from build123d import *

# Parameters (mm, degrees)
F0_R      = 4
F1_DEPTH  = 0.8
F2_R      = 2.3
F3_DEPTH  = 4.5
F4_R      = 4.5
F5_DEPTH  = 13
F6_R      = 1.5
F7_DEPTH  = 9.4
F8_R      = 1.05
F9_DEPTH  = 12.5
F10_W     = 0.4
F10_H     = 0.6
F11_DEPTH = 25
F12_COUNT = 30
F15_DEPTH = 2.5


with BuildPart() as f1:
    # F0 (on Top) → F1 (new body)
    with BuildSketch(Plane.XY):
        Circle(F0_R)
    extrude(amount=F1_DEPTH)

    # F2 (on face) → F3 (join)
    with BuildSketch(Plane.XY.offset(0.8)):
        Circle(F2_R)
    extrude(amount=F3_DEPTH)

    # F4 (on face) → F5 (join)
    with BuildSketch(Plane.XY.offset(5.3)):
        Circle(F4_R)
    extrude(amount=F5_DEPTH)

    # F6 (on face) → F7 (join)
    with BuildSketch(Plane(origin=(0, 0, 0), x_dir=(1, 0, 0), z_dir=(0, 0, -1))):
        Circle(F6_R)
    extrude(amount=F7_DEPTH)

    # F8 (on Front) → F9 (cut, symmetric)
    with BuildSketch(Plane.XZ):
        with Locations((0, 3)):
            Circle(F8_R)
    extrude(amount=F9_DEPTH, both=True, mode=Mode.SUBTRACT)


with BuildPart() as f11:
    # F10 (on face) → F11 (new body)
    with BuildSketch(Plane.XY.offset(18.3)):
        with Locations((0, 4.5)):
            Rectangle(F10_W, F10_H)
    extrude(amount=-F11_DEPTH)


with BuildPart() as f12_1:
    # F12: instance of F11
    add(f11.part.rotate(Axis((0, 0, 18.3), (0, 0, 1)), 1 * 360 / F12_COUNT))


with BuildPart() as f12_2:
    # F12: instance of F11
    add(f11.part.rotate(Axis((0, 0, 18.3), (0, 0, 1)), 2 * 360 / F12_COUNT))


with BuildPart() as f12_3:
    # F12: instance of F11
    add(f11.part.rotate(Axis((0, 0, 18.3), (0, 0, 1)), 3 * 360 / F12_COUNT))


with BuildPart() as f12_4:
    # F12: instance of F11
    add(f11.part.rotate(Axis((0, 0, 18.3), (0, 0, 1)), 4 * 360 / F12_COUNT))


with BuildPart() as f12_5:
    # F12: instance of F11
    add(f11.part.rotate(Axis((0, 0, 18.3), (0, 0, 1)), 5 * 360 / F12_COUNT))


with BuildPart() as f12_6:
    # F12: instance of F11
    add(f11.part.rotate(Axis((0, 0, 18.3), (0, 0, 1)), 6 * 360 / F12_COUNT))


with BuildPart() as f12_7:
    # F12: instance of F11
    add(f11.part.rotate(Axis((0, 0, 18.3), (0, 0, 1)), 7 * 360 / F12_COUNT))


with BuildPart() as f12_8:
    # F12: instance of F11
    add(f11.part.rotate(Axis((0, 0, 18.3), (0, 0, 1)), 8 * 360 / F12_COUNT))


with BuildPart() as f12_9:
    # F12: instance of F11
    add(f11.part.rotate(Axis((0, 0, 18.3), (0, 0, 1)), 9 * 360 / F12_COUNT))


with BuildPart() as f12_10:
    # F12: instance of F11
    add(f11.part.rotate(Axis((0, 0, 18.3), (0, 0, 1)), 10 * 360 / F12_COUNT))


with BuildPart() as f12_11:
    # F12: instance of F11
    add(f11.part.rotate(Axis((0, 0, 18.3), (0, 0, 1)), 11 * 360 / F12_COUNT))


with BuildPart() as f12_12:
    # F12: instance of F11
    add(f11.part.rotate(Axis((0, 0, 18.3), (0, 0, 1)), 12 * 360 / F12_COUNT))


with BuildPart() as f12_13:
    # F12: instance of F11
    add(f11.part.rotate(Axis((0, 0, 18.3), (0, 0, 1)), 13 * 360 / F12_COUNT))


with BuildPart() as f12_14:
    # F12: instance of F11
    add(f11.part.rotate(Axis((0, 0, 18.3), (0, 0, 1)), 14 * 360 / F12_COUNT))


with BuildPart() as f12_15:
    # F12: instance of F11
    add(f11.part.rotate(Axis((0, 0, 18.3), (0, 0, 1)), 15 * 360 / F12_COUNT))


with BuildPart() as f12_16:
    # F12: instance of F11
    add(f11.part.rotate(Axis((0, 0, 18.3), (0, 0, 1)), 16 * 360 / F12_COUNT))


with BuildPart() as f12_17:
    # F12: instance of F11
    add(f11.part.rotate(Axis((0, 0, 18.3), (0, 0, 1)), 17 * 360 / F12_COUNT))


with BuildPart() as f12_18:
    # F12: instance of F11
    add(f11.part.rotate(Axis((0, 0, 18.3), (0, 0, 1)), 18 * 360 / F12_COUNT))


with BuildPart() as f12_19:
    # F12: instance of F11
    add(f11.part.rotate(Axis((0, 0, 18.3), (0, 0, 1)), 19 * 360 / F12_COUNT))


with BuildPart() as f12_20:
    # F12: instance of F11
    add(f11.part.rotate(Axis((0, 0, 18.3), (0, 0, 1)), 20 * 360 / F12_COUNT))


with BuildPart() as f12_21:
    # F12: instance of F11
    add(f11.part.rotate(Axis((0, 0, 18.3), (0, 0, 1)), 21 * 360 / F12_COUNT))


with BuildPart() as f12_22:
    # F12: instance of F11
    add(f11.part.rotate(Axis((0, 0, 18.3), (0, 0, 1)), 22 * 360 / F12_COUNT))


with BuildPart() as f12_23:
    # F12: instance of F11
    add(f11.part.rotate(Axis((0, 0, 18.3), (0, 0, 1)), 23 * 360 / F12_COUNT))


with BuildPart() as f12_24:
    # F12: instance of F11
    add(f11.part.rotate(Axis((0, 0, 18.3), (0, 0, 1)), 24 * 360 / F12_COUNT))


with BuildPart() as f12_25:
    # F12: instance of F11
    add(f11.part.rotate(Axis((0, 0, 18.3), (0, 0, 1)), 25 * 360 / F12_COUNT))


with BuildPart() as f12_26:
    # F12: instance of F11
    add(f11.part.rotate(Axis((0, 0, 18.3), (0, 0, 1)), 26 * 360 / F12_COUNT))


with BuildPart() as f12_27:
    # F12: instance of F11
    add(f11.part.rotate(Axis((0, 0, 18.3), (0, 0, 1)), 27 * 360 / F12_COUNT))


with BuildPart() as f12_28:
    # F12: instance of F11
    add(f11.part.rotate(Axis((0, 0, 18.3), (0, 0, 1)), 28 * 360 / F12_COUNT))


with BuildPart() as f12_29:
    # F12: instance of F11
    add(f11.part.rotate(Axis((0, 0, 18.3), (0, 0, 1)), 29 * 360 / F12_COUNT))


with BuildPart() as f1_1:
    add(f1.part)

    # F13: cut F12_1, F12_2, F12_3, F12_4, F12_5, F12_6, F12_7, F12_8, F12_9, F12_10, F12_11, F12_12, F12_13, F12_14, F12_15, F12_16, F12_17, F12_18, F12_19, F12_20, F12_21, F12_22, F12_23, F12_24, F12_25, F12_26, F12_27, F12_28, F12_29, F11
    add(f12_1.part, mode=Mode.SUBTRACT)
    add(f12_2.part, mode=Mode.SUBTRACT)
    add(f12_3.part, mode=Mode.SUBTRACT)
    add(f12_4.part, mode=Mode.SUBTRACT)
    add(f12_5.part, mode=Mode.SUBTRACT)
    add(f12_6.part, mode=Mode.SUBTRACT)
    add(f12_7.part, mode=Mode.SUBTRACT)
    add(f12_8.part, mode=Mode.SUBTRACT)
    add(f12_9.part, mode=Mode.SUBTRACT)
    add(f12_10.part, mode=Mode.SUBTRACT)
    add(f12_11.part, mode=Mode.SUBTRACT)
    add(f12_12.part, mode=Mode.SUBTRACT)
    add(f12_13.part, mode=Mode.SUBTRACT)
    add(f12_14.part, mode=Mode.SUBTRACT)
    add(f12_15.part, mode=Mode.SUBTRACT)
    add(f12_16.part, mode=Mode.SUBTRACT)
    add(f12_17.part, mode=Mode.SUBTRACT)
    add(f12_18.part, mode=Mode.SUBTRACT)
    add(f12_19.part, mode=Mode.SUBTRACT)
    add(f12_20.part, mode=Mode.SUBTRACT)
    add(f12_21.part, mode=Mode.SUBTRACT)
    add(f12_22.part, mode=Mode.SUBTRACT)
    add(f12_23.part, mode=Mode.SUBTRACT)
    add(f12_24.part, mode=Mode.SUBTRACT)
    add(f12_25.part, mode=Mode.SUBTRACT)
    add(f12_26.part, mode=Mode.SUBTRACT)
    add(f12_27.part, mode=Mode.SUBTRACT)
    add(f12_28.part, mode=Mode.SUBTRACT)
    add(f12_29.part, mode=Mode.SUBTRACT)
    add(f11.part, mode=Mode.SUBTRACT)

    # F14 (on face) → F15 (join)
    with BuildSketch(Plane(origin=(0, 0, 0), x_dir=(1, 0, 0), z_dir=(0, 0, -1))):
        Polygon((-2.6927305179, -0.8780481684), (-0.5859532394, -2.7709971182), (2.1067772785, -1.8929489498), (2.6927305179, 0.8780481684), (0.5859532394, 2.7709971182), (-2.1067772785, 1.8929489498), align=None)
    extrude(amount=F15_DEPTH)


solid = f1_1.part
Can you work these out from the model? Positions are in its coordinate system, mm. A direction names the side the tool comes from. Give positions to 0.01 mm unless a question says otherwise; leave off trailing zeros. Order: outer loops, then holes, each group sorted by start corner. A loop starts at its lowest first (then second) coordinate and runs counter-clockwise, first axis right, second up. Notation, with made-up numbers: M -30,28 L -3,28 A12 ccw -3,50 Z; hole C 20.25,25 d5. An arc over 180 degrees is marked long. Use one line per item in the form item = value.
Item 1: If I drill on line 1 along Z through (x, y) = (0, 0.2); line 2 along X through (y, z) = (0.1, 3); line 3 along Z through (x, y) = (3.75, 1), over which ranges is the centre line in solid material (lowest first)? Write a range as [from, to].
Values follow:
line_1 = [-9.4, 1.95], [4.05, 18.3]
line_2 = [-2.3, -1.05], [1.05, 2.3]
line_3 = [0, 0.8], [5.3, 18.3]
Item 2: If we section it at C-C, the plane z = -7: Write out the boundary of the cut face in (x, y), and give its area (3 significant figures).
Values follow:
outline = C 0,0 d3
area = 7.07 mm^2
Item 3: If we section it at B-B, the plane z = 3: Write out the boundary of the cut face in (x, y).
Values follow:
outline = M -1.05,-2.05 L -1.05,2.05 A2.3 ccw Z; M 1.05,-2.05 A2.3 ccw 1.05,2.05 Z
Item 4: Thinking about a two-plate mould opening in X: for faces 1 (the flat face through (1.654, -1.811, -1.232)), 2 (the flat face through (1.2, 1.2, -2.5)), 3 (the cylindrical face through (0.485, -0.032, 2.068)), which applies, pulls with the +X half, pulls with the -X half, needs draft (parallel to the pull), parting line crosses it, or undercut?
Values follow:
face_1 = pulls with the +X half
face_2 = needs draft
face_3 = undercut
Item 5: Will these pins go through, and if not, where does the flat tip stop? pin 1 Ø1.7 at (x, z) = (0, 3) entering from +Y; pin 2 Ø3 at (y, z) = (-3, 3.5) entering from +X; pin 3 Ø4 at (x, z) = (0, 13.5) entering from +Y; pin 4 Ø1 at (y, z) = (3, 13.5) entering from +X.
Values follow:
pin_1 = through
pin_2 = 1.74
pin_3 = 4.5
pin_4 = 3.74
Item 6: For faces 4 (the flat face through (2, -2, 0.8)), 5 (the flat face through (0, -3, 0)), 6 (the flat face through (-1.654, 1.811, -1.232)), 7 (the flat face through (0.74, 2.34, -1.23)), 8 (the flat face through (-2.4, -0.5, -1.2)), which set-ups out of +Z, -Z, +X, -X, +Y, -Y let a thin tool reach every point of the face, with its end or its side?
Values follow:
face_4 = none
face_5 = -Z
face_6 = -Z, -X, +Y
face_7 = -Z, +X, +Y
face_8 = -Z, -X, -Y
Item 7: If we section it at A-A, the plane z = -1.5: Write out the boundary of the cut face in (x, y).
Values follow:
outline = M -2.69,0.88 L -2.11,-1.89 L 0.59,-2.77 L 2.69,-0.88 L 2.11,1.89 L -0.59,2.77 Z
